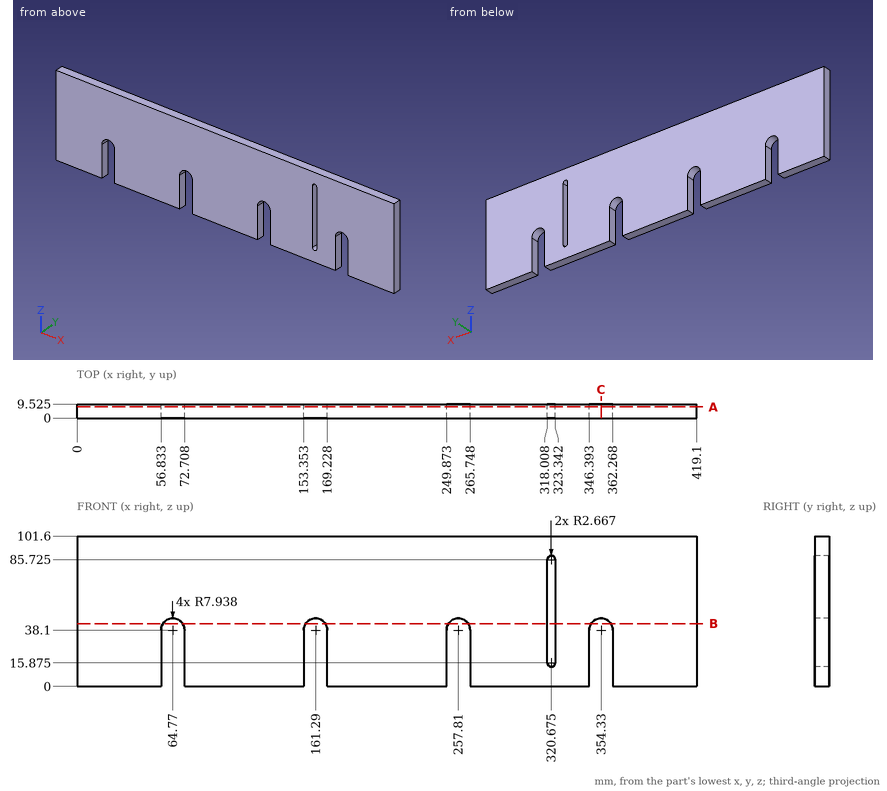
Here's the drawing with two shaded views (mm, measured from the low corner). I have some questions. Give positions to 0.01 mm unless a question says otherwise; leave off trailing zeros. Order: outer loops, then holes, each group sorted by start corner. A loop starts at its lowest first (then second) coordinate and runs counter-clockwise, first axis right, second up. Notation, with made-up numbers: (19.5, 81) - (37.5, 81) arc R17 cw to (37.5, 99) - close; hole circle Ø7 at (84.5, -21). An arc over 180 degrees is marked (long way). Use a Markdown table: item, result. Add a question column.
Q1. Please list where these lines run through material, in increasing order: line 1 along X through (y, z) = (6.5, 33); line 2 along X through (y, z) = (0.5, 39); line 3 along X through (y, z) = (6, 60.5).
Q2. If we section it at B-B on z = 42.5: Write out the boundary of the cut face in (x, y) (1 decimal), plus the area to 3 significant figures.
Q3. If we section it at C-C on x = 354.33: Write out the boundary of the cut face in (y, z) (1 decimal).
Q4. If we section it at A-A on y = 7.5: Write out the boundary of the cut face in (x, z) (1 decimal), plus the area to 3 significant figures.
Answers follow:
| question | item | result |
|---|---|---|
| 1 | line 1 | x = 0 to 56.83, 72.71 to 153.35, 169.23 to 249.87, 265.75 to 318.01, 323.34 to 346.39, 362.27 to 419.1 |
| 1 | line 2 | x = 0 to 56.88, 72.66 to 153.4, 169.18 to 249.92, 265.7 to 318.01, 323.34 to 346.44, 362.22 to 419.1 |
| 1 | line 3 | x = 0 to 318.01, 323.34 to 419.1 |
| 2 | outline | (0, 0) - (58.2, 0) - (58.2, 9.5) - (0, 9.5) - close; (71.4, 0) - (154.7, 0) - (154.7, 9.5) - (71.4, 9.5) - close; (167.9, 0) - (251.2, 0) - (251.2, 9.5) - (167.9, 9.5) - close; (264.4, 0) - (318, 0) - (318, 9.5) - (264.4, 9.5) - close; (323.3, 0) - (347.7, 0) - (347.7, 9.5) - (323.3, 9.5) - close; (360.9, 0) - (419.1, 0) - (419.1, 9.5) - (360.9, 9.5) - close |
| 2 | area | 3,440 mm^2 |
| 3 | outline | (0, 46) - (9.5, 46) - (9.5, 101.6) - (0, 101.6) - close |
| 4 | outline | (0, 0) - (56.8, 0) - (56.8, 38.1) arc R7.9 cw to (72.7, 38.1) - (72.7, 0) - (153.4, 0) - (153.4, 38.1) arc R7.9 cw to (169.2, 38.1) - (169.2, 0) - (249.9, 0) - (249.9, 38.1) arc R7.9 cw to (265.7, 38.1) - (265.7, 0) - (346.4, 0) - (346.4, 38.1) arc R7.9 cw to (362.3, 38.1) - (362.3, 0) - (419.1, 0) - (419.1, 101.6) - (0, 101.6) - close; hole (318, 15.9) arc R2.7 ccw to (323.3, 15.9) - (323.3, 85.7) arc R2.7 ccw to (318, 85.7) - close |
| 4 | area | 39,400 mm^2 |
